```python
from build123d import *

# Parameters (mm, degrees)
BOSS_EXTRUDE1_DEPTH      = 101.6
SKETCH2_R                = 4.1656
CUT_EXTRUDE1_DEPTH       = 141.047212542
SKETCH3_W                = 45.3392611
SKETCH3_H                = 95.6
CUT_EXTRUDE2_DEPTH       = 164.328230385
SKETCH5_W                = 36
SKETCH5_H                = 70
BOSS_EXTRUDE2_DEPTH      = 25
CUT_EXTRUDE3_DEPTH       = 25
FILLET1_R                = 5.08
SKETCH7_R                = 2
CUT_EXTRUDE4_DEPTH       = 139.536371578
CUT_EXTRUDE5_DEPTH       = 7.488
CUT_EXTRUDE5_DEPTH_BACK  = 44.572
SKETCH8_W                = 30.464500282
SKETCH8_H                = 15.24
BOSS_EXTRUDE3_DEPTH      = 10
BOSS_EXTRUDE4_DEPTH      = 35
BOSS_EXTRUDE4_DEPTH_BACK = 35
SKETCH11_W               = 60
SKETCH11_H               = 3
BOSS_EXTRUDE5_DEPTH      = 3
CUT_EXTRUDE6_DEPTH       = 190.450951053


with BuildPart() as part:
    # Sketch1 → Boss-Extrude1 (new body)
    with BuildSketch(Plane(origin=(0, 0, 0), x_dir=(-1, 0, 0), z_dir=(0, 0, 1))):
        with BuildLine():
            Line((57.350334268, 77.47), (29.380183448, 77.47))
            Line((29.380183448, 77.47), (29.380183448, 13.97))
            Line((29.380183448, 13.97), (16.680183448, 13.97))
            Line((16.680183448, 13.97), (16.680183448, 1.27))
            Line((16.680183448, 1.27), (19.250334268, -1.27))
            Line((19.250334268, -1.27), (19.250334268, -34.29))
            Line((19.250334268, -34.29), (16.6878, -36.83))
            Line((16.6878, -36.83), (54.810334268, -36.83))
            ThreePointArc((54.810334268, -36.83), (56.606385492, -36.086051224), (57.350334268, -34.29))
            Line((57.350334268, -34.29), (57.350334268, 77.47))
        make_face()
    extrude(amount=BOSS_EXTRUDE1_DEPTH)

    # Sketch2 → Cut-Extrude1 (cut, through all)
    with BuildSketch(Plane.XY.offset(101.6)):
        with Locations((-38.300334268, 17.78)):
            Circle(SKETCH2_R)
    extrude(amount=-CUT_EXTRUDE1_DEPTH, mode=Mode.SUBTRACT)

    # Sketch3 → Cut-Extrude2 (cut, through all)
    with BuildSketch(Plane(origin=(0, -77.47, 0), x_dir=(-1, 0, 0), z_dir=(0, -1, 0))):
        with Locations((31.680703718, -50.8)):
            Rectangle(SKETCH3_W, SKETCH3_H)
    extrude(amount=-CUT_EXTRUDE2_DEPTH, mode=Mode.SUBTRACT)

    # Sketch5 → Boss-Extrude2 (add)
    with BuildSketch(Plane(origin=(-54.350334268, 0, 0), x_dir=(0, 0, -1), z_dir=(1, 0, 0))):
        with Locations((-52.512822265, -37.765880907)):
            Rectangle(SKETCH5_W, SKETCH5_H)
    extrude(amount=BOSS_EXTRUDE2_DEPTH)

    # Sketch6 → Cut-Extrude3 (cut)
    with BuildSketch(Plane(origin=(-29.350334268, 0, 0), x_dir=(0, 0, -1), z_dir=(1, 0, 0))):
        Polygon((-67.512822265, -5.765880907), (-37.512822265, -5.765880907), (-37.512822265, -85.765880907), (-67.512822265, -85.765880907), (-67.512822265, -56.765880907), (-78.412691352, -56.765880907), (-78.412691352, -52.765880907), (-67.512822265, -52.765880907), align=None)
    extrude(amount=-CUT_EXTRUDE3_DEPTH, mode=Mode.SUBTRACT)

    # Fillet1
    fillet1_edges = [part.edges().sort_by_distance(p)[0] for p in [
        (-54.350334268, -20.32, 98.6),
        (-54.350334268, -20.32, 3),
        (-54.350334268, -37.765880907, 34.512822265),
        (-54.350334268, -27.765880907, 70.512822265),
        (-54.350334268, -64.765880907, 70.512822265),
    ]]
    fillet(fillet1_edges, radius=FILLET1_R)

    # Sketch7 → Cut-Extrude4 (cut, through all)
    with BuildSketch(Plane(origin=(0, -2.765880907, 0), x_dir=(1, 0, 0), z_dir=(0, 1, 0))):
        with Locations(Location((-49.850334378, -64.332963641, 0), (0, 0, 180))):
            Circle(SKETCH7_R)
        with Locations(Location((-35.854934378, -64.332963641, 0), (0, 0, 180))):
            Circle(SKETCH7_R)
    extrude(amount=-CUT_EXTRUDE4_DEPTH, mode=Mode.SUBTRACT)

    # Sketch8 → Cut-Extrude5 (cut, two sides: drawn at the far end of the back side and taken through both)
    with BuildSketch(Plane(origin=(0, 0, 34.512822265), x_dir=(-1, 0, 0), z_dir=(0, 0, -1)).offset(-CUT_EXTRUDE5_DEPTH_BACK)):
        with Locations((39.118084127, -15.385880813)):
            Rectangle(SKETCH8_W, SKETCH8_H)
    extrude(amount=CUT_EXTRUDE5_DEPTH + CUT_EXTRUDE5_DEPTH_BACK, mode=Mode.SUBTRACT)

    # Sketch9 → Boss-Extrude3 (add)
    with BuildSketch(Plane(origin=(0, 0, 34.512822265), x_dir=(-1, 0, 0), z_dir=(0, 0, -1))):
        Polygon((29.350334268, -2.765880907), (54.350334268, -2.765880907), (54.350334268, 12.234119093), align=None)
    extrude(amount=-BOSS_EXTRUDE3_DEPTH)

    # Sketch11 → Boss-Extrude4 (add, two sides: drawn at the far end of the back side and taken through both)
    with BuildSketch(Plane.XY.offset(50.8).offset(-BOSS_EXTRUDE4_DEPTH_BACK)):
        with Locations((-84.810334268, 35.33)):
            Rectangle(SKETCH11_W, SKETCH11_H)
    extrude(amount=BOSS_EXTRUDE4_DEPTH + BOSS_EXTRUDE4_DEPTH_BACK)

    # Sketch12 → Boss-Extrude5 (add)
    with BuildSketch(Plane.XY.offset(85.8)):
        Polygon((-114.810334268, 33.83), (-57.350334268, 33.83), (-57.350334268, 8.83), align=None)
    extrude(amount=-BOSS_EXTRUDE5_DEPTH)

    # Sketch13 → Cut-Extrude6 (cut, through all)
    with BuildSketch(Plane(origin=(0, 33.83, 0), x_dir=(-1, 0, 0), z_dir=(0, -1, 0))):
        with BuildLine():
            Line((107.269485022, -79.300000094), (67.264485022, -79.300000094))
            ThreePointArc((67.264485022, -79.300000094), (65.764485022, -77.800000094), (67.264485022, -76.300000094))
            Line((67.264485022, -76.300000094), (107.269485022, -76.300000094))
            ThreePointArc((107.269485022, -76.300000094), (108.769485022, -77.800000094), (107.269485022, -79.300000094))
        make_face()
        with BuildLine():
            Line((107.269485022, -22.302400094), (67.264485022, -22.302400094))
            ThreePointArc((67.264485022, -22.302400094), (65.764485022, -20.802400094), (67.264485022, -19.302400094))
            Line((67.264485022, -19.302400094), (107.269485022, -19.302400094))
            ThreePointArc((107.269485022, -19.302400094), (108.769485022, -20.802400094), (107.269485022, -22.302400094))
        make_face()
    extrude(amount=-CUT_EXTRUDE6_DEPTH, mode=Mode.SUBTRACT)


solid = part.part
```
CAD build for the part. Positions are in the model's coordinates, mm. A direction names the side the tool comes from. Round coordinates to 2 decimals unless told otherwise and drop trailing zeros. Loops run counter-clockwise (first coordinate to the right, second up) from the corner with the lowest first, then second, coordinate; pieces in that order, holes last. Notation, with made-up numbers: M 84.5,22.25 L 97.5,22.25 A22 cw 97.5,36.25 Z; hole C 39.25,38 d1. An arc over 180 degrees is marked long. Return JSON: item names as keys, results as strings. Group by question number.
(1) Saw through at D-D, the plane z = 77.8. List the corners of the cut face in (x, y).
(2) Mould opens along Z. For faces 5 (the flat face through (-19.25, 18, 1)), 6 (the flat face through (-41, -21, 101.6)), 7 (the flat face through (-39, -65, 70.513)) say: +Z half, -Z half, draft (parallel to the pull), parting line (faces both ways), or undercut.
(3) Saw through at C-C, the plane y = 17.78. List the corners of the cut face in (x, z), and give its area (3 significant figures).
(4) Tool access for faces 1 (the cylindrical face through (-52.9, -5.23, 72.04)), 2 (the flat face through (-43, -23.006, 36)), 3 (the flat face through (-53.1, -2.766, 33.5)), 4 (the flat face through (-88, 35, 79.3)): list every direction of +Z, -Z, +X, -X, +Y, -Y with a clear straight run to the whole face (end or side of a thin tool).
(5) Saw through at B-B, the plane z = 40.5. List the corners of the cut face in (x, y).
(6) Saw through at A-A, the plane x = -81.5. List the corners of the cut face in (y, z), and give its area (3 significant figures).
(7) Drop flat-ended pins along their axis: P1, Ø6.5, axis at x = -38.5, z = 72.5, coming from the -Y side; P2, Ø0.9, axis at y = 18, z = 1, coming from the +X side; P3, Ø1, axis at y = -6, z = 70.5, coming from the +X side; P4, Ø3, axis at x = -49.85, z = 64.33, coming from the -Y side. Give the stop position or say it passes through.
(8) Wall check: probe 1 along Z at (x, y) = (-49, 4); probe 2 along Z at (x, y) = (-30.5, -23.5); probe 3 along Z at (x, y) = (-47, 29). Give the ranges that are in metal, low to high. Write a range as [from, to].
Answer list:
{
 "1": {"outline": "M -114.81,33.83 L -108.77,33.83 L -108.77,36.83 L -114.81,36.83 Z; M -65.76,33.83 L -57.35,33.83 L -57.35,-77.47 L -54.35,-77.47 L -54.35,36.83 L -65.76,36.83 Z"},
 "2": {"face 5": "draft", "face 6": "+Z half", "face 7": "undercut"},
 "3": {"outline": "M -77.92,82.8 L -57.35,82.8 L -57.35,0 L -42.47,0 L -42.47,3 L -49.27,3 A5.08 cw -54.35,8.08 L -54.35,93.52 A5.08 cw -49.27,98.6 L -42.47,98.6 L -42.47,101.6 L -57.35,101.6 L -57.35,85.8 L -77.92,85.8 Z; M -34.13,0 L -19.25,0 L -19.25,3 L -34.13,3 Z; M -34.13,98.6 L -19.25,98.6 L -19.25,101.6 L -34.13,101.6 Z", "area": "538 mm2"},
 "4": {"face 1": "+X, +Y, -Y", "face 2": "+X", "face 3": "+X, +Y", "face 4": "+Y, -Y"},
 "5": {"outline": "M -114.81,33.83 L -57.35,33.83 L -57.35,-77.47 L -54.35,-77.47 L -54.35,-5.77 L -29.35,-5.77 L -29.35,-2.77 L -54.35,12.23 L -54.35,36.83 L -114.81,36.83 Z"},
 "6": {"outline": "M 19.34,82.8 L 33.83,82.8 L 33.83,79.3 L 36.83,79.3 L 36.83,85.8 L 19.34,85.8 Z; M 33.83,15.8 L 36.83,15.8 L 36.83,19.3 L 33.83,19.3 Z; M 33.83,22.3 L 36.83,22.3 L 36.83,76.3 L 33.83,76.3 Z", "area": "235 mm2"},
 "7": {"P1": "y = -72.77", "P2": "x = -19.25", "P3": "x = -29.35", "P4": "through"},
 "8": {"probe 1": "[0, 3], [34.51, 44.51], [98.6, 101.6]", "probe 2": "[0, 3], [34.51, 37.51], [67.51, 70.51], [98.6, 101.6]", "probe 3": "[0, 3], [98.6, 101.6]"}
}
